CAD build for the part. Positions are in the model's coordinates, mm. Face numbers are marked on the shaded views. Coordinates: 2 decimals unless noted, no trailing zeros. Loops run counter-clockwise (first coordinate to the right, second up) from the corner with the lowest first, then second, coordinate; pieces in that order, holes last. Notation, with made-up numbers: (23, 84) - (35, 84) arc R31 ccw to (35, 113) - close; hole circle Ø5 at (57.5, -1.75). An arc over 180 degrees is marked (long way). Put each result on its own line as item: value.
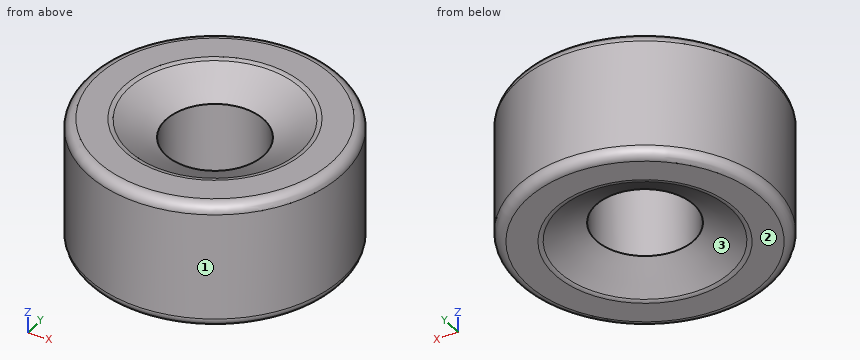
Autodesk Inventor part; units mm, degrees
ref_plane "Work Plane1" through (0, 0, 6.5) normal (0, 0, 1) x (1, 0, 0)
ref_plane "YZ Plane" through (0, 0, 0) normal (1, 0, 0) x (0, 1, 0)
ref_plane "XZ Plane" through (0, 0, 0) normal (0, 1, 0) x (-1, 0, 0)
sketch "Sketch1" plane through (0, 0, 0) normal (0, 0, 1) x (1, 0, 0)
  circle A0 centre (0, 0) radius 13
  dimension "d0" = 26
extrude "Extrusion1" add sketch "Sketch1" along normal blind 13
sketch "Sketch2" plane through (0, 0, 13) normal (0, 0, 1) x (1, 0, 0)
  circle A0 centre (0, 0) radius 13
hole "Hole1" at (0, 0, 13) direction (0, 0, -1) diameter 10 end through all
sketch "Sketch3" plane through (0, 0, 0) normal (0, 1, 0) x (-1, 0, 0)
  line L0 (0, 13) -> (0, 0)
  line L1 (-5, 13) -> (5, 13)
  line L2 (13, 13) -> (-13, 13)
  line L3 (5, 0) -> (5, 13)
  line L4 (5, 11) -> (9, 13)
  line L5 (9, 13) -> (5, 13)
  line L6 (5, 13) -> (5, 11)
  dimension "d10" = 2
  dimension "d11" = 4
revolve "Revolution1" cut sketch "Sketch3" angle 360 about axis through (0, 0, 13) along (0, 0, -1)
ref_plane "Work Plane1" through (0, 0, 6.5) normal (0, 0, 1) x (1, 0, 0)
mirror "Mirror1" about plane through (0, 0, 6.5) normal (0, 0, 1) of "Revolution1"
fillet "Fillet1" radius 1 4 edges at (-13, 0, 0) (9, 0, 0) (-13, 0, 13) (9, 0, 13)
properties part number "Wheel"
Q1. Pin check, flat tips, straight feed: pin 1 Ø12 at (x, y) = (-8, 2) entering from -Z; pin 2 Ø3 at (y, z) = (-7.5, 4.5) entering from -X; pin 3 Ø6 at (x, z) = (5.5, 5.5) entering from -Y. Stop position of each tip, or through.
Determined:
pin 1: z = 0
pin 2: x = -11.53
pin 3: y = -12.76
Q2. Slice it at D-D, the plane z = 11.5. Give the cut face in (x, y), then the cut area to 3 significant figures.
Determined:
outline: circle Ø26 at (0, 0); hole circle Ø12 at (0, 0)
area: 418 mm2
Q3. Wall check: L1, parallel to Y at x = 0, z = 5.5; L2, parallel to X at y = -2.5, z = 3.25. Give the ranges that are in metal, low to high. Write a range as from..to.
Determined:
L1: -13..-5, 5..13
L2: -12.76..-4.33, 4.33..12.76
Q4. Slice it at A-A, the plane x = 0. Give the cut face in (y, z).
Determined:
outline: (-13, 1) arc R1 ccw to (-12, 0) - (-9.24, 0) arc R1 ccw to (-8.79, 0.11) - (-5, 2) - (-5, 11) - (-8.79, 12.89) arc R1 ccw to (-9.24, 13) - (-12, 13) arc R1 ccw to (-13, 12) - close; (5, 2) - (8.79, 0.11) arc R1 ccw to (9.24, 0) - (12, 0) arc R1 ccw to (13, 1) - (13, 12) arc R1 ccw to (12, 13) - (9.24, 13) arc R1 ccw to (8.79, 12.89) - (5, 11) - close
Q5. Slice it at C-C, the plane z = 7.75. Give the cut face in (x, y), then the cut area to 3 significant figures.
Determined:
outline: circle Ø26 at (0, 0); hole circle Ø10 at (0, 0)
area: 452 mm2
Q6. Mould opens along Y. For the marked faces 1, 2 and 3 say: +Y half, -Y half, draft (parallel to the pull), parting line (faces both ways), or undercut.
Determined:
face 1: parting line
face 2: draft
face 3: undercut
